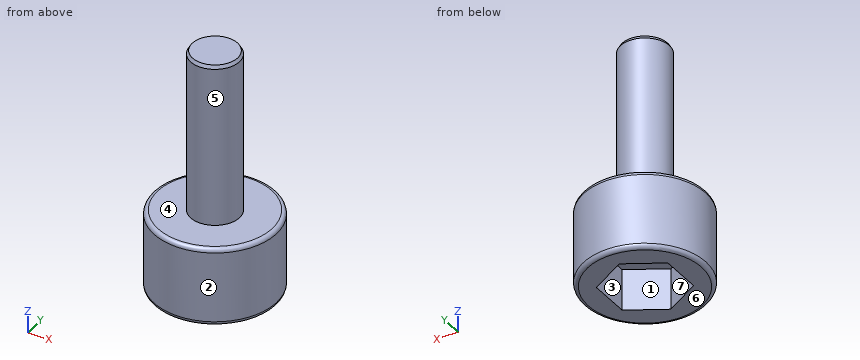
```python
from build123d import *

# Parameters (mm, degrees)
CUT_EXTRUDE1_DEPTH  = 2.54
SKETCH3_R           = 1.5
BOSS_EXTRUDE1_DEPTH = 10
CHAMFER1_SIZE       = 0.2
CHAMFER1_SIZE2      = 0.115470054


with BuildPart() as part:
    # Sketch1 → Revolve1 (revolve)
    with BuildSketch(Plane(origin=(0, 0, 0), x_dir=(1, 0, 0), z_dir=(0, 1, 0))):
        with BuildLine():
            Line((0, 0), (3.5, 0))
            ThreePointArc((3.5, 0), (3.679605122, -0.074394878), (3.754, -0.254))
            Line((3.754, -0.254), (3.754, -4.572))
            ThreePointArc((3.754, -4.572), (3.679605122, -4.751605122), (3.5, -4.826))
            Line((3.5, -4.826), (0, -4.826))
            Line((0, -4.826), (0, 0))
        make_face()
    revolve(axis=Axis((0, 0, 0), (0, 0, -1)))

    # Sketch2 → Cut-Extrude1 (cut)
    with BuildSketch(Plane(origin=(0, 0, 0), x_dir=(-1, 0, 0), z_dir=(0, 0, -1))):
        Polygon((0, 2.55), (-2.20836478, 1.275), (-2.20836478, -1.275), (0, -2.55), (2.20836478, -1.275), (2.20836478, 1.275), align=None)
    extrude(amount=-CUT_EXTRUDE1_DEPTH, mode=Mode.SUBTRACT)

    # Sketch3 → Boss-Extrude1 (add)
    with BuildSketch(Plane.XY.offset(4.826)):
        Circle(SKETCH3_R)
    extrude(amount=BOSS_EXTRUDE1_DEPTH)

    # Chamfer1
    chamfer1_edges = [part.edges().sort_by_distance(p)[0] for p in [
        (-1.5, 0, 14.826),
    ]]
    chamfer1_side = [part.faces().sort_by_distance(p)[0] for p in [
        (-1.5, 0, 9.826),
    ]]
    chamfer(chamfer1_edges, length=CHAMFER1_SIZE, length2=CHAMFER1_SIZE2, reference=chamfer1_side[0])


solid = part.part
```
The listing builds one solid part. Answer for the finished solid, in the listing's coordinates (mm). Face numbers are marked on the shaded views. A direction names the side the tool comes from. Round coordinates to 2 decimals unless told otherwise and drop trailing zeros. Loops run counter-clockwise (first coordinate to the right, second up) from the corner with the lowest first, then second, coordinate; pieces in that order, holes last.
Q1. Section B-B, the plane y = 0 is taken. Determine the outline of the cut face in (x, z).
Q2. For a pull along X with two mould halves and no side action, classify the marked faces 1, 2, 3 and 4 as released by +X, released by -X, zero draft, split by the parting line, or undercut.
Q3. Section C-C, the plane z = 5 is taken. Determine the outline of the cut face in (x, y), then the cut area to 3 significant figures.
Q4. Which of the six approach directions +Z, -Z, +X, -X, +Y, -Y give full straight-line access (tool end or side, diameter ignored) to the marked faces 5, 6 and 7?
Q5. Given pin 1 Ø4 at (x, z) = (0.5, 10.5) entering from -Y; pin 2 Ø2 at (x, z) = (1.5, 13) entering from -Y; pin 3 Ø1.3 at (x, y) = (0, 1) entering from -Z, each flat-ended and moving along its own axis, determine where each tip first touches the part or whether it passes through.
Q6. Find the intervals of material crossed by line 1 (Z direction, x = 3, y = 1.75); line 2 (Z direction, x = -1.5, y = -1.25); line 3 (Y direction, x = -0.5, z = 2.5), in increasing order.
Q7. Section A-A, the plane z = 1.25 is taken. Determine the outline of the cut face in (x, y) (3 decimals).
Completed:
1. outline: (-3.75, 0.25) arc R0.25 ccw to (-3.5, 0) - (-2.21, 0) - (-2.21, 2.54) - (2.21, 2.54) - (2.21, 0) - (3.5, 0) arc R0.25 ccw to (3.75, 0.25) - (3.75, 4.57) arc R0.25 ccw to (3.5, 4.83) - (1.5, 4.83) - (1.5, 14.63) - (1.38, 14.83) - (-1.38, 14.83) - (-1.5, 14.63) - (-1.5, 4.83) - (-3.5, 4.83) arc R0.25 ccw to (-3.75, 4.57) - close
2. face 1: undercut
2. face 2: split by the parting line
2. face 3: undercut
2. face 4: zero draft
3. outline: circle Ø3 at (0, 0)
3. area: 7.07 mm2
4. face 5: +Z
4. face 6: -Z, +X, -X, +Y, -Y
4. face 7: -Z
5. pin 1: stops at y = -1.5
5. pin 2: stops at y = -1.41
5. pin 3: stops at z = 2.54
6. line 1: z = 0 to 4.83
6. line 2: z = 2.54 to 4.83
6. line 3: y = -3.72 to -2.26, 2.26 to 3.72
7. outline: circle Ø7.508 at (0, 0); hole (-2.208, -1.275) - (0, -2.55) - (2.208, -1.275) - (2.208, 1.275) - (0, 2.55) - (-2.208, 1.275) - close
